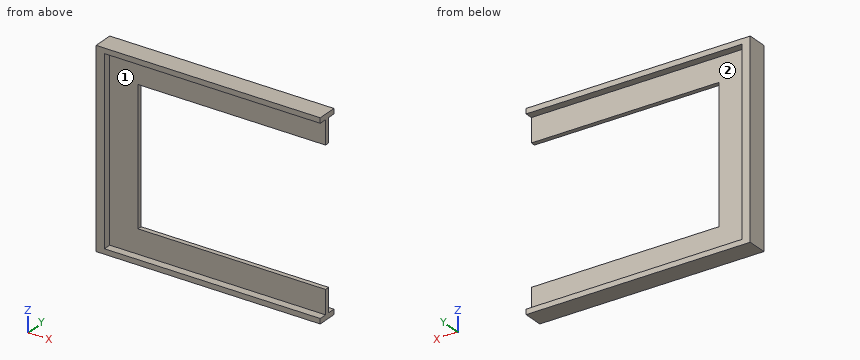
from build123d import *

# Parameters (mm, degrees)
BOSS_EXTRUDE1_DEPTH      = 1.4
BOSS_EXTRUDE2_DEPTH      = 2.4
BOSS_EXTRUDE2_DEPTH_BACK = 3.8


with BuildPart() as part:
    # Sketch1 → Boss-Extrude1 (new body)
    with BuildSketch(Plane(origin=(0, 0, 0), x_dir=(1, 0, 0), z_dir=(0, 1, 0))):
        Polygon((0, 0), (5.4, 0), (5.4, -7), (5.4, -9), (-58.4, -9), (-61.4, -9), (-64.4, -9), (-64.4, 51), (-61.4, 51), (-58.4, 51), (5.4, 51), (5.4, 49), (5.4, 42), (0, 42), (-53, 42), (-53, 0), align=None)
    extrude(amount=BOSS_EXTRUDE1_DEPTH)

    # Sketch2 → Boss-Extrude2 (add, two sides: drawn at the far end of the back side and taken through both)
    with BuildSketch(Plane(origin=(0, 1.4, 0), x_dir=(1, 0, 0), z_dir=(0, 1, 0)).offset(-BOSS_EXTRUDE2_DEPTH_BACK)):
        Polygon((-64.4, 51), (5.4, 51), (5.4, 49.4), (-61.8, 49.4), (-61.8, -7.4), (5.4, -7.4), (5.4, -9), (-64.4, -9), align=None)
    extrude(amount=BOSS_EXTRUDE2_DEPTH + BOSS_EXTRUDE2_DEPTH_BACK)


solid = part.part
Design review of the part built by this model. Coordinates are the model's own, in mm. Face numbers are marked on the shaded views. A direction names the side the tool comes from. Round coordinates to 2 decimals unless told otherwise and drop trailing zeros. Loops run counter-clockwise (first coordinate to the right, second up) from the corner with the lowest first, then second, coordinate; pieces in that order, holes last. Notation, with made-up numbers: (13, 25) - (28, 25) arc R24 ccw to (28, 43) - close; hole circle Ø10 at (54.5, -37). An arc over 180 degrees is marked (long way). One line per item, written item: value. Start each with the question number.
1) To check wall thickness, follow L1, parallel to Z at x = -22.5, y = -2; L2, parallel to X at y = -1.5, z = -36; L3, parallel to Y at x = -35.5, z = 4. State the ranges of each line that lie inside material, in increasing order. Write a range as from..to.
2) Insertion check: pin 1 Ø3 at (x, z) = (-24, -43.5) entering from +Y; pin 2 Ø0.7 at (y, z) = (-1.5, -9) entering from +X; pin 3 Ø1.5 at (x, z) = (-52.5, -32.5) entering from -Y. Each pin has a flat end and moves straight along its axis. Give the tip position at first contact, or say it passes through.
3) For the marked faces 1 and 2, list the 3-axis set-ups (+Z, -Z, +X, -X, +Y, -Y) from which the entire face can be reached by the end or side of a thin tool; tool diameter is ignored.
4) Consider section A-A on x = -48. Give the boundary of the cut face in (y, z), then the cut area to 3 significant figures.
5) Consider section D-D on z = 5.5. Give the boundary of the cut face in (x, y).
6) Consider section B-B on x = -58. Give the boundary of the cut face in (y, z).
7) Consider section C-C on y = 2.25. Give the boundary of the cut face in (x, z), then the cut area to 3 significant figures.
Reported:
1. L1: z = -51..-49.4, 7.4..9
1. L2: x = -64.4..-61.8
1. L3: y = 0..1.4
2. pin 1: stops at y = 1.4
2. pin 2: stops at x = -61.8
2. pin 3: stops at y = 0
3. face 1: +X, -Y
3. face 2: +X, +Y
4. outline: (-2.4, -51) - (3.8, -51) - (3.8, -49.4) - (1.4, -49.4) - (1.4, -42) - (0, -42) - (0, -49.4) - (-2.4, -49.4) - close; (-2.4, 7.4) - (0, 7.4) - (0, 0) - (1.4, 0) - (1.4, 7.4) - (3.8, 7.4) - (3.8, 9) - (-2.4, 9) - close
4. area: 40.6 mm^2
5. outline: (-64.4, -2.4) - (-61.8, -2.4) - (-61.8, 0) - (5.4, 0) - (5.4, 1.4) - (-61.8, 1.4) - (-61.8, 3.8) - (-64.4, 3.8) - close
6. outline: (-2.4, -51) - (3.8, -51) - (3.8, -49.4) - (1.4, -49.4) - (1.4, 7.4) - (3.8, 7.4) - (3.8, 9) - (-2.4, 9) - (-2.4, 7.4) - (0, 7.4) - (0, -49.4) - (-2.4, -49.4) - close
7. outline: (-64.4, -51) - (5.4, -51) - (5.4, -49.4) - (-61.8, -49.4) - (-61.8, 7.4) - (5.4, 7.4) - (5.4, 9) - (-64.4, 9) - close
7. area: 371 mm^2
